```python
from build123d import *

# Parameters (mm, degrees)
OUTLINESKETCH2_W                           = 50
OUTLINESKETCH2_H                           = 55.4
OUTLINESKETCH2_R                           = 2
OUTLINEBOSS_EXTRUDE1_DEPTH                 = 18.05
BUILDPLATECUTOUTSKETCH1_W                  = 49
BUILDPLATECUTOUTSKETCH1_H                  = 46
BUILDPLATECUTOUTCUT_EXTRUDE7_DEPTH         = 7
MICROSWITCHSKETCH9_W                       = 13.05
MICROSWITCHSKETCH9_H                       = 12.05
MICROSWITCHCUT_EXTRUDE6_DEPTH              = 6.3
MICROSWITCHMOUNTINGHOLESSKETCH10_R         = 1.5
MICROSWITCHMOUNTINGHOLESCUT_EXTRUDE4_DEPTH = 3.1
CABLECUTCUT_EXTRUDE5_DEPTH                 = 76.59340249
HEATMATCUTSKETCH3_W                        = 34
HEATMATCUTSKETCH3_H                        = 31
HEATMATCUT_EXTRUDE8_DEPTH                  = 2
BALLJOINTCUT_EXTRUDE9_DEPTH                = 6.05
CHAMFER1_SIZE                              = 7
CHAMFER1_SIZE2                             = 18.475
CHAMFER2_SIZE                              = 6
CHAMFER2_SIZE2                             = 18.475


with BuildPart() as part:
    # OutlineSketch2 → OutlineBoss-Extrude1 (new body)
    with BuildSketch(Plane(origin=(0, 0, 0), x_dir=(1, 0, 0), z_dir=(0, 1, 0))):
        with Locations((25, 27.7)):
            Rectangle(OUTLINESKETCH2_W, OUTLINESKETCH2_H)
        with Locations(Location((42, 5, 0), (0, 0, 270))):
            Circle(OUTLINESKETCH2_R, mode=Mode.SUBTRACT)
    extrude(amount=OUTLINEBOSS_EXTRUDE1_DEPTH)

    # BuildPlateCutoutSketch1 → BuildPlateCutoutCut-Extrude7 (cut)
    with BuildSketch(Plane(origin=(0, 18.05, 0), x_dir=(1, 0, 0), z_dir=(0, 1, 0))):
        with Locations((24.5, 23)):
            Rectangle(BUILDPLATECUTOUTSKETCH1_W, BUILDPLATECUTOUTSKETCH1_H)
    extrude(amount=-BUILDPLATECUTOUTCUT_EXTRUDE7_DEPTH, mode=Mode.SUBTRACT)

    # MicroSwitchSketch9 → MicroSwitchCut-Extrude6 (cut)
    with BuildSketch(Plane(origin=(0, 0, -55.4), x_dir=(-1, 0, 0), z_dir=(0, 0, -1))):
        with Locations((-25, 12.025)):
            Rectangle(MICROSWITCHSKETCH9_W, MICROSWITCHSKETCH9_H)
    extrude(amount=-MICROSWITCHCUT_EXTRUDE6_DEPTH, mode=Mode.SUBTRACT)

    # MicroSwitchMountingHolesSketch10 → MicroSwitchMountingHolesCut-Extrude4 (cut)
    with BuildSketch(Plane(origin=(0, 0, -49.1), x_dir=(-1, 0, 0), z_dir=(0, 0, -1))):
        with Locations((-28.175, 13)):
            Circle(MICROSWITCHMOUNTINGHOLESSKETCH10_R)
        with Locations((-21.825, 13)):
            Circle(MICROSWITCHMOUNTINGHOLESSKETCH10_R)
    extrude(amount=-MICROSWITCHMOUNTINGHOLESCUT_EXTRUDE4_DEPTH, mode=Mode.SUBTRACT)

    # CableCutSketch11 → CableCutCut-Extrude5 (cut, through all)
    with BuildSketch(Plane(origin=(0, 6, 0), x_dir=(1, 0, 0), z_dir=(0, 1, 0))):
        Polygon((24.125, 55.4), (24.125, 53.65), (23.125, 53.65), (23.125, 51.9), (26.875, 51.9), (26.875, 53.65), (25.875, 53.65), (25.875, 55.4), align=None)
    extrude(amount=-CABLECUTCUT_EXTRUDE5_DEPTH, mode=Mode.SUBTRACT)

    # HeatMatCutSketch3 → HeatMatCut-Extrude8 (cut)
    with BuildSketch(Plane(origin=(0, 11.05, 0), x_dir=(1, 0, 0), z_dir=(0, 1, 0))):
        with Locations((17, 15.5)):
            Rectangle(HEATMATCUTSKETCH3_W, HEATMATCUTSKETCH3_H)
    extrude(amount=-HEATMATCUT_EXTRUDE8_DEPTH, mode=Mode.SUBTRACT)

    # BallJointCutoutSketch4 → BallJointCut-Extrude9 (cut)
    with BuildSketch(Plane.XZ):
        with BuildLine():
            Line((25.020895194, 0), (50, 0))
            Line((50, 0), (50, -20.788920166))
            ThreePointArc((50, -20.788920166), (30.677417203, -18.604746187), (25.020895194, 0))
        make_face()
    extrude(amount=-BALLJOINTCUT_EXTRUDE9_DEPTH, mode=Mode.SUBTRACT)

    # Chamfer1
    chamfer1_edges = [part.edges().sort_by_distance(p)[0] for p in [
        (0, 18.05, -50.7),
    ]]
    chamfer1_side = [part.faces().sort_by_distance(p)[0] for p in [
        (0, 6.03362055, -31.38491972),
    ]]
    chamfer(chamfer1_edges, length=CHAMFER1_SIZE, length2=CHAMFER1_SIZE2, reference=chamfer1_side[0])

    # Chamfer2
    chamfer2_edges = [part.edges().sort_by_distance(p)[0] for p in [
        (50, 18.05, -27.7),
    ]]
    chamfer2_side = [part.faces().sort_by_distance(p)[0] for p in [
        (50, 9.888235373, -30.189792368),
    ]]
    chamfer(chamfer2_edges, length=CHAMFER2_SIZE, length2=CHAMFER2_SIZE2, reference=chamfer2_side[0])


solid = part.part
```
The model under review builds one solid part; all positions refer to its coordinate system, in mm. A direction names the side the tool comes from. Round coordinates to 2 decimals unless told otherwise and drop trailing zeros. Order: outer loops, then holes, each group sorted by start corner. A loop starts at its lowest first (then second) coordinate and runs counter-clockwise, first axis right, second up. Notation, with made-up numbers: (9, -3) - (27, -3) arc R18 ccw to (27, 9) - close; hole circle Ø6 at (83, 63). An arc over 180 degrees is marked (long way). Answer in a Markdown table with one row per item.
(1) Take a section at A-A on z = -5. Write out the cut boundary in (x, y).
Result set:
| item | result |
|---|---|
| outline | (0, 0) - (24.3, 0) - (24.3, 6.05) - (40, 6.05) - (40, 11.05) - (34, 11.05) - (34, 9.05) - (0, 9.05) - close; (44, 6.05) - (50, 6.05) - (50, 12.05) - (49, 12.37) - (49, 11.05) - (44, 11.05) - close |
(2) Mouldability with a two-part tool opening along X and no side actions: class faces 4 (the face through (50, 6, -33)), 5 (the face through (30, 11.05, -34)), 6 (the face through (20.394, 13.451, -47.572)), 7 (the face through (0, 5, -27)) as released by +X, released by -X, zero draft, split by the parting line, or undercut.
Result set:
| item | result |
|---|---|
| face 4 | released by +X |
| face 5 | zero draft |
| face 6 | undercut |
| face 7 | released by -X |
(3) For line 1 (Y direction, x = 40, z = -41.5); line 2 (Z direction, x = 27.5, y = 10.5); line 3 (Y direction, x = 4.5, z = -9), list the stretches that pass through material, from the lowest coordinate up. Write a range as from..to.
Result set:
| item | result |
|---|---|
| line 1 | y = 0..11.05 |
| line 2 | z = -49.1..-31 |
| line 3 | y = 0..9.05 |
(4) Take a section at B-B on x = 42. Write out the cut boundary in (y, z), plus the area to 3 significant figures.
Result set:
| item | result |
|---|---|
| outline | (0, -55.4) - (14.65, -55.4) - (14.65, -46) - (11.05, -46) - (11.05, -7) - (6.05, -7) - (6.05, -22.7) - (0, -22.7) - close; (6.05, -3) - (11.05, -3) - (11.05, 0) - (6.05, 0) - close |
| area | 489 mm2 |
(5) Take a section at D-D on y = 13. Write out the cut boundary in (x, z) (3 decimals), plus the area to 3 significant figures.
Result set:
| item | result |
|---|---|
| outline | (5.147, -55.4) - (18.475, -55.4) - (18.475, -49.1) - (20.325, -49.1) - (20.325, -46) - (5.147, -46) - close; (23.325, -49.1) - (26.675, -49.1) - (26.675, -46) - (23.325, -46) - close; (29.675, -49.1) - (31.525, -49.1) - (31.525, -55.4) - (47.075, -55.4) - (47.075, -46) - (29.675, -46) - close |
| area | 293 mm2 |
(6) Machinability: for faces 1 (the face through (25.875, 3, -55)), 2 (the face through (49, 12, -23)), 3 (the face through (18.475, 12, -52)), which of the approach directions +Z, -Z, +X, -X, +Y, -Y give a long, thin tool a straight path to every point of the face, cutting with its end or side? Answer none if there is none.
Result set:
| item | result |
|---|---|
| face 1 | -Z, +Y, -Y |
| face 2 | +Z, -X, +Y |
| face 3 | -Z, +Y |
(7) Clearance check with flat-ended pins moving along their axes: P1, Ø0.6, axis at x = 23, y = 10.5, coming from the +Z side; P2, Ø1, axis at y = 10.5, z = -19, coming from the -X side; P3, Ø3.5, axis at x = 23, y = 11.5, coming from the -Z side. State where each tip first meets the part, or that it passes through.
Result set:
| item | result |
|---|---|
| P1 | stops at z = -31 |
| P2 | stops at x = 34 |
| P3 | stops at z = -49.1 |
(8) Take a section at C-C on z = -28.5. Write out the cut boundary in (x, y), plus the area to 3 significant figures.
Result set:
| item | result |
|---|---|
| outline | (0, 0) - (50, 0) - (50, 12.05) - (49, 12.37) - (49, 11.05) - (34, 11.05) - (34, 9.05) - (0, 9.05) - close |
| area | 486 mm2 |
